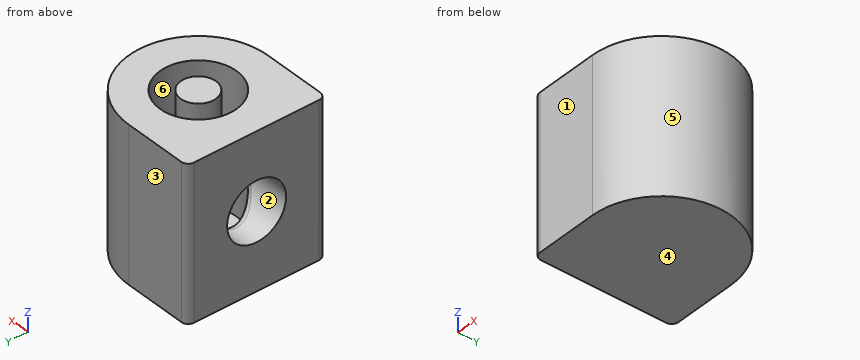
from build123d import *

# Parameters (mm, degrees)
F0_R     = 5.5
F1_DEPTH = 22
F0_R_2   = 2.54
F2_DEPTH = 2
F3_R     = 4.25
F4_DEPTH = 10
F5_DEPTH = 22
F6_R     = 1


with BuildPart() as f1:
    # F0 (on Top) → F1 (new body)
    with BuildSketch(Plane.XY):
        with BuildLine():
            Line((-10, -10), (0, -10))
            ThreePointArc((0, -10), (10, 0), (0, 10))
            Line((0, 10), (-10, 10))
            Line((-10, 10), (-10, -10))
        make_face()
        Circle(F0_R, mode=Mode.SUBTRACT)
    extrude(amount=F1_DEPTH)

    # F0 (on Top) → F2 (join)
    with BuildSketch(Plane.XY):
        Circle(F0_R)
        Circle(F0_R_2, mode=Mode.SUBTRACT)
    extrude(amount=F2_DEPTH)

    # F3 (on face) → F4 (cut)
    with BuildSketch(Plane(origin=(-10, 0, 0), x_dir=(0, -1, 0), z_dir=(-1, 0, 0))):
        with Locations((0, 11)):
            Circle(F3_R)
    extrude(amount=-F4_DEPTH, mode=Mode.SUBTRACT)

    # F0 (on Top) → F5 (join)
    with BuildSketch(Plane.XY):
        Circle(F0_R_2)
    extrude(amount=F5_DEPTH)

    # F6
    f6_edges = [f1.edges().sort_by_distance(p)[0] for p in [
        (-10, -10, 11),
        (-10, 10, 11),
        (-3.49106, 4.25, 11),
    ]]
    fillet(f6_edges, radius=F6_R)


solid = f1.part
Here's how the part is built. I have some questions about the finished solid (model axes, mm). Face numbers are marked on the shaded views. A direction names the side the tool comes from. Round coordinates to 2 decimals unless told otherwise and drop trailing zeros. Write each loop counter-clockwise with the first axis right and the second up, starting at its lowest first coordinate (ties: lowest second). Pieces come first, ordered by that corner, then holes.
1. I need wall thicknesses on L1, parallel to Y at x = -1.25, z = 4.75; L2, parallel to X at y = -1.75, z = 16; L3, parallel to Y at x = -7.5, z = 11. Which ranges of each line are inside material? Lowest first, please.
2. Suppose I cut it at C-C (x = 4.5). List the corners of the cut face in (y, z) for me, and give its area (3 significant figures).
3. For the marked faces 5 and 6, which set-ups out of +Z, -Z, +X, -X, +Y, -Y let a thin tool reach every point of the face, with its end or its side?
4. If we mould it in two halves opening along Y, with no side actions, what happens to the marked faces 1, 2, 3 and 4? For each: released by +Y, released by -Y, zero draft, split by the parting line, or undercut.
5. Will this pin go through, and if not, where does the flat tip stop? pin 1 Ø6 at (x, z) = (4, 16) entering from -Y.
6. Suppose I cut it at A-A (z = 19.25). List the corners of the cut face in (x, y) for me, and give its area (3 significant figures).
7. Suppose I cut it at B-B (y = -5). List the corners of the cut face in (x, z) for me.
Answer sheet:
1. L1: y = -10 to -5.36, -2.21 to 2.21, 5.36 to 10
1. L2: x = -10 to -5.21, -1.84 to 1.84, 5.21 to 9.85
1. L3: y = -10 to -4.25, 4.25 to 10
2. outline: (-8.93, 0) - (8.93, 0) - (8.93, 22) - (3.16, 22) - (3.16, 2) - (-3.16, 2) - (-3.16, 22) - (-8.93, 22) - close
2. area: 266 mm2
3. face 5: +Z, -Z, +X
3. face 6: +Z
4. face 1: released by -Y
4. face 2: undercut
4. face 3: released by +Y
4. face 4: zero draft
5. pin 1: stops at y = -9.95
6. outline: (-10, -9) arc R1 ccw to (-9, -10) - (0, -10) arc R10 ccw to (0, 10) - (-9, 10) arc R1 ccw to (-10, 9) - close; circle Ø5.08 at (0, 0); hole circle Ø11 at (0, 0)
6. area: 282 mm2
7. outline: (-10, 0) - (8.66, 0) - (8.66, 22) - (2.29, 22) - (2.29, 2) - (-2.29, 2) - (-2.29, 22) - (-10, 22) - close
